Model file for the job. Use its own axes, mm. Face numbers are marked on the shaded views. Coordinates: 2 decimals unless noted, no trailing zeros. Loops run counter-clockwise (first coordinate to the right, second up) from the corner with the lowest first, then second, coordinate; pieces in that order, holes last.
from build123d import *

# Parameters (mm, degrees)
SKETCH_2_R               = 41
SKETCH_2_R_2             = 30
EXTRUDE_1_DEPTH          = 4
SKETCH_3_R               = 1.5
CUT_EXTRUDE_1_DEPTH      = 59.120564347
CUT_EXTRUDE_2_DEPTH      = 3
PATTERN_CIRCULAR_1_COUNT = 24
SKETCH_5_R               = 1.5
CUT_EXTRUDE_3_DEPTH      = 59.120564347
CUT_EXTRUDE_4_DEPTH      = 3
PATTERN_CIRCULAR_2_COUNT = 24


with BuildPart() as part:
    # 草图2 → 凸台-拉伸1 (new body)
    with BuildSketch(Plane(origin=(0, 0, 0), x_dir=(1, 0, 0), z_dir=(0, 1, 0))):
        with Locations(Location((0, 0, 0), (0, 0, 270))):
            Circle(SKETCH_2_R)
        with Locations(Location((0, 0, 0), (0, 0, 270))):
            Circle(SKETCH_2_R_2, mode=Mode.SUBTRACT)
    extrude(amount=EXTRUDE_1_DEPTH)

    # 草图3 → 切除-拉伸1 (cut, through all)
    with BuildSketch(Plane(origin=(0, 4, 0), x_dir=(1, 0, 0), z_dir=(0, 1, 0))):
        with Locations(Location((0, 37, 0), (0, 0, 270))):
            Circle(SKETCH_3_R)
    cut_extrude_1 = extrude(amount=-CUT_EXTRUDE_1_DEPTH, mode=Mode.SUBTRACT)

    # 草图4 → 切除-拉伸2 (cut)
    with BuildSketch(Plane(origin=(0, 4, 0), x_dir=(1, 0, 0), z_dir=(0, 1, 0))):
        Polygon((3.175426481, 37), (1.58771324, 39.75), (-1.58771324, 39.75), (-3.175426481, 37), (-1.58771324, 34.25), (1.58771324, 34.25), align=None)
    cut_extrude_2 = extrude(amount=-CUT_EXTRUDE_2_DEPTH, mode=Mode.SUBTRACT)

    # 阵列(圆周)1: 切除-拉伸1, 切除-拉伸2 ×24 about axis, 16 skipped
    pattern_circular_1_axis = Axis((0, 4, 0), (0, 1, 0))
    add([cut_extrude_1.rotate(pattern_circular_1_axis, i * 360 / PATTERN_CIRCULAR_1_COUNT) for i in range(1, PATTERN_CIRCULAR_1_COUNT) if i not in (1, 2, 4, 5, 7, 8, 10, 11, 13, 14, 16, 17, 19, 20, 22, 23)], mode=Mode.SUBTRACT)
    add([cut_extrude_2.rotate(pattern_circular_1_axis, i * 360 / PATTERN_CIRCULAR_1_COUNT) for i in range(1, PATTERN_CIRCULAR_1_COUNT) if i not in (1, 2, 4, 5, 7, 8, 10, 11, 13, 14, 16, 17, 19, 20, 22, 23)], mode=Mode.SUBTRACT)

    # 草图5 → 切除-拉伸3 (cut, through all)
    with BuildSketch(Plane.XZ):
        with Locations(Location((13.393920133, 32.335783638, 0), (0, 0, 270))):
            Circle(SKETCH_5_R)
    cut_extrude_3 = extrude(amount=-CUT_EXTRUDE_3_DEPTH, mode=Mode.SUBTRACT)

    # 草图6 → 切除-拉伸4 (cut)
    with BuildSketch(Plane.XZ):
        Polygon((12.178737028, 29.402072106), (15.326997295, 29.816548433), (16.5421804, 32.750259965), (14.609103238, 35.26949517), (11.460842971, 34.855018843), (10.245659866, 31.921307311), align=None)
    cut_extrude_4 = extrude(amount=-CUT_EXTRUDE_4_DEPTH, mode=Mode.SUBTRACT)

    # 阵列(圆周)2: 切除-拉伸3, 切除-拉伸4 ×24 about axis, 16 skipped
    pattern_circular_2_axis = Axis((0, 0, 0), (0, 1, 0))
    add([cut_extrude_3.rotate(pattern_circular_2_axis, i * 360 / PATTERN_CIRCULAR_2_COUNT) for i in range(1, PATTERN_CIRCULAR_2_COUNT) if i not in (1, 2, 4, 5, 7, 8, 10, 11, 13, 14, 16, 17, 19, 20, 22, 23)], mode=Mode.SUBTRACT)
    add([cut_extrude_4.rotate(pattern_circular_2_axis, i * 360 / PATTERN_CIRCULAR_2_COUNT) for i in range(1, PATTERN_CIRCULAR_2_COUNT) if i not in (1, 2, 4, 5, 7, 8, 10, 11, 13, 14, 16, 17, 19, 20, 22, 23)], mode=Mode.SUBTRACT)


solid = part.part
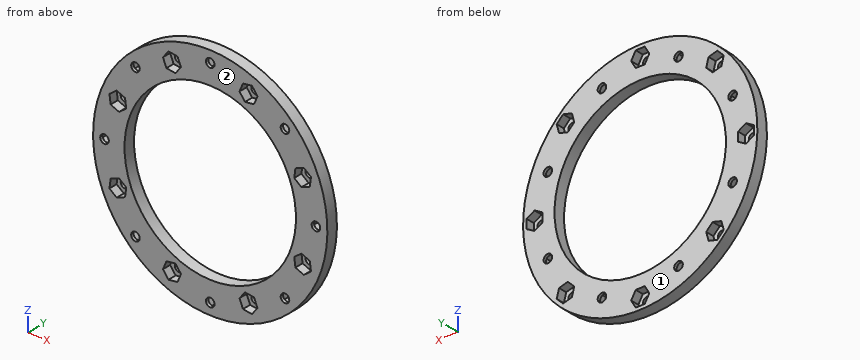
Q1. Drill centre lines: line 1 (Z direction, x = 1, y = 1.6); line 2 (X direction, y = 0.8, z = 34); line 3 (X direction, y = 0.35, z = -13). Where is each one in solid material? Low to high.
Answers:
line 1: z = -40.99 to -39.75, -34.25 to -29.98, 29.98 to 34.25, 39.75 to 40.99
line 2: x = -22.91 to -15.58, -11.11 to 11.11, 15.58 to 22.91
line 3: x = -38.88 to -35.06, -29.51 to -27.04, 27.04 to 29.51, 35.06 to 38.88
Q2. Slice it at B-B (z = 5). List the corners of the cut face in (x, y), and give its area (3 significant figures).
Answers:
outline: (-40.69, 0) - (-29.58, 0) - (-29.58, 4) - (-40.69, 4) - close; (29.58, 0) - (40.69, 0) - (40.69, 4) - (29.58, 4) - close
area: 88.9 mm2
Q3. Slice it at D-D (x = -22). List the corners of the cut face in (y, z).
Answers:
outline: (0, -34.6) - (4, -34.6) - (4, -20.4) - (0, -20.4) - close; (0, 20.4) - (4, 20.4) - (4, 34.6) - (0, 34.6) - close
Q4. Slice it at A-A (x = 0). List the corners of the cut face in (y, z).
Answers:
outline: (0, -41) - (4, -41) - (4, -39.75) - (1, -39.75) - (1, -38.5) - (0, -38.5) - close; (0, -35.5) - (1, -35.5) - (1, -34.25) - (4, -34.25) - (4, -30) - (0, -30) - close; (0, 30) - (4, 30) - (4, 34.25) - (1, 34.25) - (1, 35.5) - (0, 35.5) - close; (0, 38.5) - (1, 38.5) - (1, 39.75) - (4, 39.75) - (4, 41) - (0, 41) - close
Q5. Mould opens along Y. For the marked faces 1 and 2 say: +Y half, -Y half, draft (parallel to the pull), parting line (faces both ways), or undercut.
Answers:
face 1: +Y half
face 2: -Y half
Q6. Flat gauge pins, fed straight in: P1, Ø1, axis at y = 3.5, z = -9, coming from the -X side; P2, Ø3.5, axis at x = -37, z = 0, coming from the +Y side; P3, Ø1.5, axis at x = 24, y = 2.5, coming from the +Z side. Where does each tip first touch, or does it go through?
Answers:
P1: stops at x = -40.11
P2: stops at y = 1
P3: stops at z = 33.77
Q7. Slice it at C-C (y = 1.8). Count the separate pieces of the cut face and the enclosed holes in it, and give its area (3 significant figures).
Answers:
separate pieces: 1
enclosed holes: 17
area: 2,030 mm2
